from build123d import *

# Parameters (mm, degrees)
SKETCH_1_W          = 78
SKETCH_1_H          = 180
EXTRUDE_1_DEPTH     = 4
CUT_EXTRUDE_1_DEPTH = 4
SKETCH_6_W          = 8
SKETCH_6_H          = 8
EXTRUDE_2_DEPTH     = 4
SKETCH_7_R          = 2
CUT_EXTRUDE_2_DEPTH = 10


with BuildPart() as part:
    # 草图1 → 凸台-拉伸1 (new body)
    with BuildSketch(Plane.XY):
        with Locations((-4, -57.5)):
            Rectangle(SKETCH_1_W, SKETCH_1_H)
    extrude(amount=EXTRUDE_1_DEPTH)

    # 草图2 → 切除-拉伸1 (cut)
    with BuildSketch(Plane.XY.offset(4)):
        Polygon((-31.5, -147.5), (-31.5, -143.5), (-32.9, -143.5), (-32.9, -140.9), (-31.5, -140.9), (-31.5, -138.9), (-28.5, -138.9), (-28.5, -140.9), (-27.1, -140.9), (-27.1, -143.5), (-28.5, -143.5), (-28.5, -147.5), align=None)
        Polygon((23.5, -147.5), (20.5, -147.5), (20.5, -143.5), (19.1, -143.5), (19.1, -140.9), (20.5, -140.9), (20.5, -138.9), (23.5, -138.9), (23.5, -140.9), (24.9, -140.9), (24.9, -143.5), (23.5, -143.5), align=None)
        Polygon((-5.5, -147.5), (-5.5, -143.5), (-6.9, -143.5), (-6.9, -140.9), (-5.5, -140.9), (-5.5, -138.9), (-2.5, -138.9), (-2.5, -140.9), (-1.1, -140.9), (-1.1, -143.5), (-2.5, -143.5), (-2.5, -147.5), align=None)
    extrude(amount=-CUT_EXTRUDE_1_DEPTH, mode=Mode.SUBTRACT)

    # 草图6 → 凸台-拉伸2 (add)
    with BuildSketch(Plane.XY.offset(4)):
        with Locations((-17, -147.5)):
            Rectangle(SKETCH_6_W, SKETCH_6_H)
        with Locations((9, -147.5)):
            Rectangle(SKETCH_6_W, SKETCH_6_H)
    extrude(amount=-EXTRUDE_2_DEPTH)

    # 草图7 → 切除-拉伸2 (cut)
    with BuildSketch(Plane(origin=(0, 0, 0), x_dir=(-1, 0, 0), z_dir=(0, 0, -1))):
        with Locations((-29, 26.5)):
            Circle(SKETCH_7_R)
        with Locations((-29, -43.5)):
            Circle(SKETCH_7_R)
        with Locations((-29, -113.5)):
            Circle(SKETCH_7_R)
        with Locations((37, -43.5)):
            Circle(SKETCH_7_R)
        with Locations((37, -113.5)):
            Circle(SKETCH_7_R)
        with Locations((37, 26.5)):
            Circle(SKETCH_7_R)
        Polygon((29, 18.5), (-16.384156611, 18.5), (29, -77.769423114), align=None)
        Polygon((-21, -105.5), (-21, -9.230576886), (24.384156611, -105.5), align=None)
    extrude(amount=-CUT_EXTRUDE_2_DEPTH, mode=Mode.SUBTRACT)


solid = part.part
Input: part model. Units: mm. Frame: model coordinates. A direction names the side the tool comes from. Round coordinates to 2 decimals unless told otherwise and drop trailing zeros. Order: outer loops, then holes, each group sorted by start corner. A loop starts at its lowest first (then second) coordinate and runs counter-clockwise, first axis right, second up.
1. Set-up query: faces 4 (the face through (-25, -147.5, 2)), 5 (the face through (-38.075, -111.814, 1.972)), 6 (the face through (-30, -138.9, 2)), 7 (the face through (-17, -151.5, 2)), 8 (the face through (29, -147.5, 2)). Return all of +Z, -Z, +X, -X, +Y, -Y with unobstructed straight access to the full face (end or side cutting, diameter ignored); none if empty.
The answers:
face 4: +Z, -Z, -X, -Y
face 5: +Z, -Z
face 6: +Z, -Z, -Y
face 7: +Z, -Z, +X, -X, -Y
face 8: +Z, -Z, +X, -Y
2. Mould query, pull axis Y, two halves, no side actions, for faces 1 (the face through (13, -150, 2)), 2 (the face through (17, -147.5, 2)), 3 (the face through (-5.99, -28.96, 1.97)). Classes: released by +Y, released by -Y, zero draft, split by the parting line, or undercut.
The answers:
face 1: zero draft
face 2: released by -Y
face 3: undercut
3. Cut plane C-C, the plane y = -92. Output: boundary loops of the cut face in (x, z).
The answers:
outline: (-43, 0) - (-18.02, 0) - (-18.02, 4) - (-43, 4) - close; (21, 0) - (35, 0) - (35, 4) - (21, 4) - close
4. Material intervals for line 1 (Y direction, x = 29, z = 2.5); line 2 (Y direction, x = -11.5, z = 0.65); line 3 (Y direction, x = -7.5, z = 0.6), sorted ascending.
The answers:
line 1: y = -147.5 to -115.5, -111.5 to -45.5, -41.5 to 24.5, 28.5 to 32.5
line 2: y = -147.5 to -105.5, -78.17 to -40.65, 18.5 to 32.5
line 3: y = -147.5 to -105.5, -69.69 to -32.16, 18.5 to 32.5
5. Cut plane B-B, the plane x = 29. Output: boundary loops of the cut face in (y, z), then the cut area to 3 significant figures.
The answers:
outline: (-147.5, 0) - (-115.5, 0) - (-115.5, 4) - (-147.5, 4) - close; (-111.5, 0) - (-45.5, 0) - (-45.5, 4) - (-111.5, 4) - close; (-41.5, 0) - (24.5, 0) - (24.5, 4) - (-41.5, 4) - close; (28.5, 0) - (32.5, 0) - (32.5, 4) - (28.5, 4) - close
area: 672 mm2
6. Cut plane D-D, the plane y = -43.5. Output: boundary loops of the cut face in (x, z), then the cut area to 3 significant figures.
The answers:
outline: (-43, 0) - (-39, 0) - (-39, 4) - (-43, 4) - close; (-35, 0) - (-29, 0) - (-29, 4) - (-35, 4) - close; (-12.84, 0) - (4.84, 0) - (4.84, 4) - (-12.84, 4) - close; (21, 0) - (27, 0) - (27, 4) - (21, 4) - close; (31, 0) - (35, 0) - (35, 4) - (31, 4) - close
area: 151 mm2
7. Cut plane A-A, the plane y = 26.5. Output: boundary loops of the cut face in (x, z), then the cut area to 3 significant figures.
The answers:
outline: (-43, 0) - (-39, 0) - (-39, 4) - (-43, 4) - close; (-35, 0) - (27, 0) - (27, 4) - (-35, 4) - close; (31, 0) - (35, 0) - (35, 4) - (31, 4) - close
area: 280 mm2
8. Pin query (flat end, axial travel): P1, Ø0.9, axis at x = 22, z = 1.5, coming from the -Y side; P2, Ø3, axis at x = -37, y = -113.5, coming from the +Z side. Return the tip coordinate at first contact, or that it passes through.
The answers:
P1: stops at y = -138.9
P2: passes through
